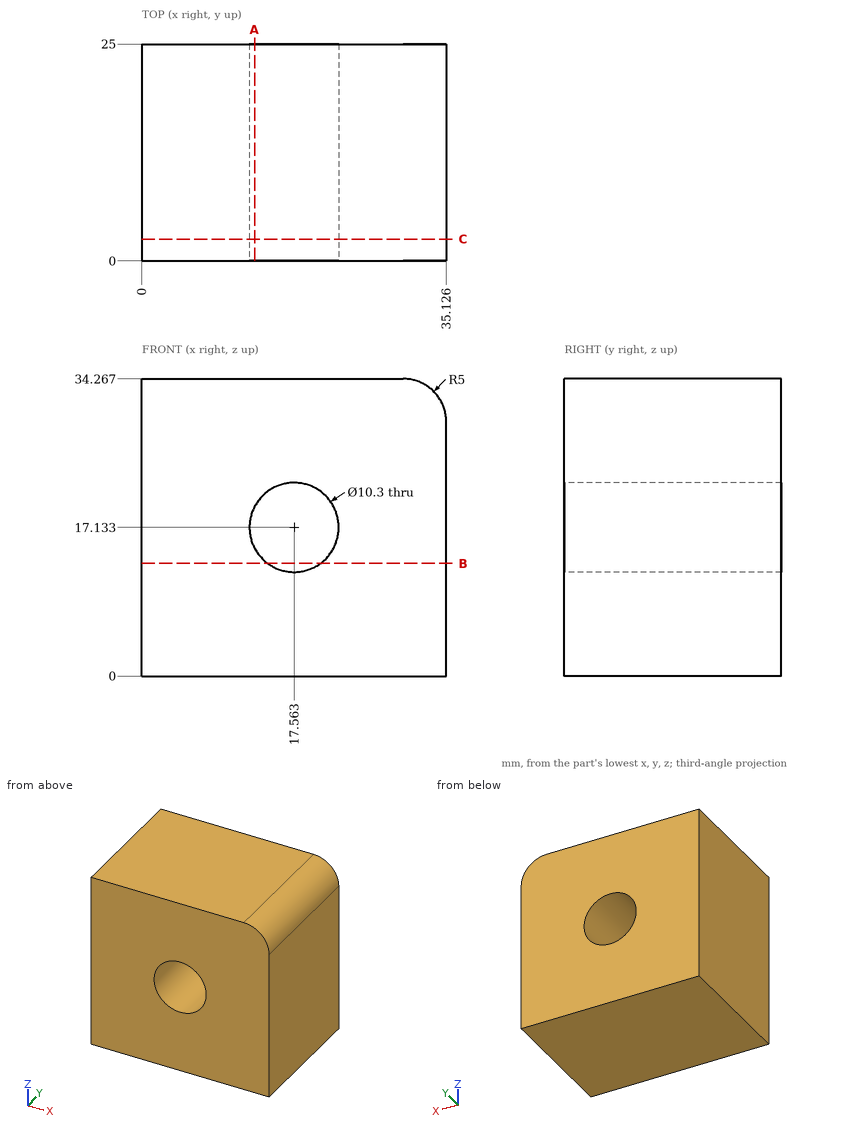
Study the drawing (mm; zero at the part's minimum x, y, z) and answer. Coordinates: 2 decimals unless noted, no trailing zeros. Loops run counter-clockwise (first coordinate to the right, second up) from the corner with the lowest first, then second, coordinate; pieces in that order, holes last. Notation, with made-up numbers: M 67.25,4.25 L 87.25,4.25 A16 ccw 87.25,13.25 Z; hole C 42,-2.5 d3. An arc over 180 degrees is marked long. Answer as a JSON object with one key per item and string values. Group by question number.
Item 1: Section A-A (x = 13) is taken. Write down the section's boundary in (y, z) (1 decimal), and give its area (3 significant figures).
Item 2: Section B-B (z = 13) is taken. Write down the section's boundary in (x, y) (1 decimal).
Item 3: Consider L1, parallel to Z at x = 17.5, y = 18.5; L2, parallel to X at y = 11, z = 13 (1 decimal); L3, parallel to Z at x = 19, y = 6. Determine where each line is inside the solid, lowest interval first.
Item 4: Each of these flat-tipped pins is pushed along its axis until it touches: P1, Ø4, axis at x = 7.5, y = 17, coming from the -Z side; P2, Ø8, axis at x = 17.56, z = 17.13, coming from the +Y side. Where does it stop, or does it pass through?
Item 5: Section C-C (y = 2.5) is taken. Write down the section's boundary in (x, z), and give its area (4 significant figures).
Solved:
{
 "1": {"outline": "M 0,0 L 25,0 L 25,14.7 L 0,14.7 Z; M 0,19.5 L 25,19.5 L 25,34.3 L 0,34.3 Z", "area": "737 mm2"},
 "2": {"outline": "M 0,0 L 14.5,0 L 14.5,25 L 0,25 Z; M 20.6,0 L 35.1,0 L 35.1,25 L 20.6,25 Z"},
 "3": {"L1": "z = 0 to 11.98, 22.28 to 34.27", "L2": "x = 0 to 14.5, 20.6 to 35.1", "L3": "z = 0 to 12.19, 22.08 to 34.27"},
 "4": {"P1": "stops at z = 0", "P2": "passes through"},
 "5": {"outline": "M 0,0 L 35.13,0 L 35.13,29.27 A5 ccw 30.13,34.27 L 0,34.27 Z; hole C 17.56,17.13 d10.3", "area": "1,115 mm2"}
}
